Source: CAD feature listing. Evaluate the final solid. Frame: model axes, mm. Face numbers are marked on the shaded views. Give positions to 0.01 mm unless a question says otherwise; leave off trailing zeros. Order: outer loops, then holes, each group sorted by start corner. A loop starts at its lowest first (then second) coordinate and runs counter-clockwise, first axis right, second up. Notation, with made-up numbers: (37.5, 86.5) - (56.5, 86.5) arc R26 ccw to (56.5, 123.5) - close; hole circle Ø11 at (74.25, 11.5). An arc over 180 degrees is marked (long way). Answer as CSV lines item,"result".
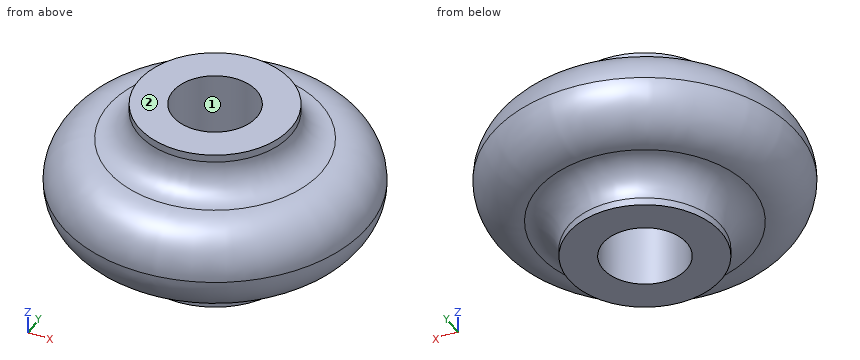
```python
from build123d import *

# Parameters (mm, degrees)
F0_R     = 5
F0_R_2   = 2.75
F1_DEPTH = 5.5
F0_R_3   = 10
F2_DEPTH = 3
F3_R     = 2.99999
F4_R     = 2


# Not quite as in the source:
# - a fillet or chamfer is up to 0.001 mm smaller than in the source, because OpenCascade refuses the exact size


with BuildPart() as f1:
    # F0 (on Top) → F1 (new body, symmetric)
    with BuildSketch(Plane.XY):
        Circle(F0_R)
        Circle(F0_R_2, mode=Mode.SUBTRACT)
    extrude(amount=F1_DEPTH, both=True)

    # F0 (on Top) → F2 (join, symmetric)
    with BuildSketch(Plane.XY):
        Circle(F0_R_3)
        Circle(F0_R, mode=Mode.SUBTRACT)
    extrude(amount=F2_DEPTH, both=True)

    # F3 (radius 3 in the source; OpenCascade refuses exactly that, so slightly less here)
    f3_edges = [f1.edges().sort_by_distance(p)[0] for p in [
        (-10, 0, 3),
        (-10, 0, -3),
    ]]
    fillet(f3_edges, radius=F3_R)

    # F4
    f4_edges = [f1.edges().sort_by_distance(p)[0] for p in [
        (-5, 0, 3),
        (-5, 0, -3),
    ]]
    fillet(f4_edges, radius=F4_R)


solid = f1.part
```
(1) Ray query, line 1 (Y direction, x = 0, z = -3.5); line 2 (X direction, y = 1.25, z = 1); line 3 (Y direction, x = 1, z = -3.5). Return the intervals inside material, ascending. Write a range as from..to.
Completed:
line 1,"-5.68..-2.75, 2.75..5.68"
line 2,"-9.75..-2.45, 2.45..9.75"
line 3,"-5.59..-2.56, 2.56..5.59"
(2) Contact query for flat-ended pins moving along their axis: pin 1 (12 mm diameter, centred on x = 0.5, y = -5, fed in from +Z); pin 2 (6 mm diameter, centred on y = -3, z = -3.5, fed in from -X); pin 3 (4 mm diameter, centred on x = 5.5, z = -1, fed in from +Y); pin 4 (5 mm diameter, centred on x = 8, y = -4, fed in from +Z). Output: stop coordinate, or through.
Completed:
pin 1,"z = 5.5"
pin 2,"x = -9.75"
pin 3,"y = 9.3"
pin 4,"z = 3.08"
(3) Cut plane D-D (z = -3.5). Return loops of the section in (x, y), then the cut area to 3 significant figures.
Completed:
outline,"circle Ø11.35 at (0, 0); hole circle Ø5.5 at (0, 0)"
area,"77.5 mm²"
(4) Cut plane C-C (z = -0.5). Return loops of the section in (x, y).
Completed:
outline,"circle Ø19.92 at (0, 0); hole circle Ø5.5 at (0, 0)"
(5) Mould query, pull axis Y, two halves, no side actions, for the marked faces 1 and 2. Classes: released by +Y, released by -Y, zero draft, split by the parting line, or undercut.
Completed:
face 1,"undercut"
face 2,"zero draft"
